from build123d import *

# Parameters (mm, degrees)
SKETCH1_R           = 11.5
BOSS_EXTRUDE1_DEPTH = 1.6825
SKETCH1_5_R         = 9.625
CUT_EXTRUDE1_DEPTH  = 3.6825
SKETCH1_6_R         = 13.75
BOSS_EXTRUDE2_DEPTH = 1.62
SKETCH1_7_R         = 9.625
CUT_EXTRUDE2_DEPTH  = 14.62
SKETCH7_R           = 0.625
CUT_EXTRUDE5_DEPTH  = 58.62
CIRPATTERN1_COUNT   = 20
SKETCH1_8_R         = 11.5
BOSS_EXTRUDE3_DEPTH = 1.19
SKETCH1_9_R         = 9.625
CUT_EXTRUDE6_DEPTH  = 19.19
SCALE1_SCALE        = 25.4


with BuildPart() as part:
    # Sketch1 → Boss-Extrude1 (new body)
    with BuildSketch(Plane.XY):
        Circle(SKETCH1_R)
    extrude(amount=BOSS_EXTRUDE1_DEPTH)

    # Sketch1_5 → Cut-Extrude1 (cut)
    with BuildSketch(Plane.XY):
        Circle(SKETCH1_5_R)
    extrude(amount=CUT_EXTRUDE1_DEPTH, mode=Mode.SUBTRACT)

    # Sketch1_6 → Boss-Extrude2 (add)
    with BuildSketch(Plane.XY):
        Circle(SKETCH1_6_R)
    extrude(amount=BOSS_EXTRUDE2_DEPTH)

    # Sketch1_7 → Cut-Extrude2 (cut)
    with BuildSketch(Plane.XY):
        Circle(SKETCH1_7_R)
    extrude(amount=CUT_EXTRUDE2_DEPTH, mode=Mode.SUBTRACT)

    # Sketch7 → Cut-Extrude5 (cut)
    with BuildSketch(Plane.XY):
        with Locations((0, 12.5)):
            Circle(SKETCH7_R)
    cut_extrude5 = extrude(amount=CUT_EXTRUDE5_DEPTH, mode=Mode.SUBTRACT)

    # CirPattern1: Cut-Extrude5 ×20 about axis
    cirpattern1_axis = Axis((0, 0, 0), (0, 0, 1))
    for i in range(1, CIRPATTERN1_COUNT):
        add(cut_extrude5.rotate(cirpattern1_axis, i * 360 / CIRPATTERN1_COUNT), mode=Mode.SUBTRACT)

    # Sketch1_8 → Boss-Extrude3 (add)
    with BuildSketch(Plane.XY):
        Circle(SKETCH1_8_R)
    extrude(amount=-BOSS_EXTRUDE3_DEPTH)

    # Sketch1_9 → Cut-Extrude6 (cut)
    with BuildSketch(Plane.XY):
        Circle(SKETCH1_9_R)
    extrude(amount=-CUT_EXTRUDE6_DEPTH, mode=Mode.SUBTRACT)


with BuildPart() as part_1:
    # Scale1: scaled about (0, 0, 0.477928167)
    add(part.part.scale(SCALE1_SCALE).moved(Location((0, 0, -11.661447275))))


solid = part_1.part
The model under review builds one solid part; all positions refer to its coordinate system, in mm. A direction names the side the tool comes from. Coordinates: 2 decimals unless noted, no trailing zeros. Write each loop counter-clockwise with the first axis right and the second up, starting at its lowest first coordinate (ties: lowest second). Pieces come first, ordered by that corner, then holes. Notation, with made-up numbers: (72.25, 77) - (87.25, 77) arc R17 cw to (87.25, 86) - close; hole circle Ø4 at (59.25, 53.25). An arc over 180 degrees is marked (long way). Answer as a JSON object with one key per item and string values. Group by question number.
1. Add section B-B (x = -24). Give the boundary of the cut face in (y, z), plus the area to 3 significant figures.
2. Clearance check with flat-ended pins moving along their axes: pin 1 Ø2 at (y, z) = (-247, -25.5) entering from -X; pin 2 Ø1.5 at (y, z) = (189, 8.5) entering from -X; pin 3 Ø1 at (x, z) = (200.5, -33) entering from +Y. State where each tip first meets the part, or that it passes through.
3. Add section C-C (z = -29). Give the boundary of the cut face in (x, y) (3 decimals), plus the area to 3 significant figures.
4. Add section A-A (y = 0). Give the boundary of the cut face in (x, z) (3 decimals), plus the area to 3 significant figures.
5. Add section D-D (x = -190.5). Give the boundary of the cut face in (y, z).
6. Machinability: for faces 1 (the face through (76, -283, 29.487)), 2 (the face through (-180.3, 242.3, 8.6)), which of the approach directions +Z, -Z, +X, -X, +Y, -Y give a long, thin tool a straight path to every point of the face, cutting with its end or side? Answer none if there is none.
7. To check wall thickness, follow probe 1 along Y at (x, z) = (-298, 5); probe 2 along X at (y, z) = (295.5, 16); probe 3 along Y at (x, z) = (2.5, -38). State the ranges of each line that lie inside material, in increasing order.
8. Mouldability with a two-part tool opening along X and no side actions: class faces 3 (the face through (-75.711, -340.945, 8.625)), 4 (the face through (194.912, 243.324, 8.625)), 5 (the face through (76, -283, -11.661)) as pulls with the +X half, pulls with the -X half, needs draft (parallel to the pull), parting line crosses it, or undercut.
Findings:
{
 "1": {"outline": "(-348.42, -11.66) - (-291.11, -11.66) - (-291.11, -41.89) - (-243.29, -41.89) - (-243.29, 31.07) - (-291.11, 31.07) - (-291.11, 29.49) - (-348.42, 29.49) - close; (243.29, -41.89) - (291.11, -41.89) - (291.11, -11.66) - (348.42, -11.66) - (348.42, 29.49) - (291.11, 29.49) - (291.11, 31.07) - (243.29, 31.07) - close", "area": "11,700 mm²"},
 "2": {"pin 1": "x = -157.5", "pin 2": "x = -294.17", "pin 3": "y = 212.89"},
 "3": {"outline": "circle Ø584.2 at (0, 0); hole circle Ø488.95 at (0, 0)", "area": "80,300 mm²"},
 "4": {"outline": "(-349.25, -11.661) - (-333.375, -11.661) - (-333.375, 29.487) - (-349.25, 29.487) - close; (-301.625, -11.661) - (-292.1, -11.661) - (-292.1, -41.887) - (-244.475, -41.887) - (-244.475, 31.074) - (-292.1, 31.074) - (-292.1, 29.487) - (-301.625, 29.487) - close; (244.475, -41.887) - (292.1, -41.887) - (292.1, -11.661) - (301.625, -11.661) - (301.625, 29.487) - (292.1, 29.487) - (292.1, 31.074) - (244.475, 31.074) - close; (333.375, -11.661) - (349.25, -11.661) - (349.25, 29.487) - (333.375, 29.487) - close", "area": "9,040 mm²"},
 "5": {"outline": "(-292.72, -11.66) - (-272.26, -11.66) - (-272.26, 29.49) - (-292.72, 29.49) - close; (-241.47, -11.66) - (-221.43, -11.66) - (-221.43, -41.89) - (-153.22, -41.89) - (-153.22, 31.07) - (-221.43, 31.07) - (-221.43, 29.49) - (-241.47, 29.49) - close; (153.22, -41.89) - (221.43, -41.89) - (221.43, -11.66) - (241.47, -11.66) - (241.47, 29.49) - (221.43, 29.49) - (221.43, 31.07) - (153.22, 31.07) - close; (272.26, -11.66) - (292.72, -11.66) - (292.72, 29.49) - (272.26, 29.49) - close"},
 "6": {"face 1": "+Z", "face 2": "+Z, -Z"},
 "7": {"probe 1": "-182.13 to -113.49, -82.74 to 82.74, 113.49 to 182.13", "probe 2": "-186.16 to -112.61, -83.61 to 83.61, 112.61 to 186.16", "probe 3": "-292.09 to -244.46, 244.46 to 292.09"},
 "8": {"face 3": "parting line crosses it", "face 4": "undercut", "face 5": "needs draft"}
}
